Source: CAD feature listing. Evaluate the final solid. Frame: model axes, mm. A direction names the side the tool comes from. Give positions to 0.01 mm unless a question says otherwise; leave off trailing zeros. Order: outer loops, then holes, each group sorted by start corner. A loop starts at its lowest first (then second) coordinate and runs counter-clockwise, first axis right, second up. Notation, with made-up numbers: M 80.5,-18.75 L 89.5,-18.75 A28 ccw 89.5,8.25 Z; hole C 20.25,-22.5 d3. An arc over 180 degrees is marked long. Use CSV: the item, a comma, the result in double quotes. Start each with the question number.
Item 1: Section query A-A on y = 71. Return loops of the section in (x, z), and give its area (3 significant figures).
Item 2: Section query D-D on z = -6. Return loops of the section in (x, y).
Item 3: Ray query, probe 1 along X at (y, z) = (65, 1); probe 2 along Z at (x, y) = (-9, 83.5); probe 3 along Y at (x, z) = (-10, -19.25). Return the intervals inside material, ascending. Write a range as from..to.
Item 4: Section query B-B on z = 1. Return loops of the section in (x, y).
Item 5: Access query for faces 1 (the face through (-12, 62, 0)), 2 (the face through (4.62, 86.46, 1.48)), 3 (the face through (-11.717, 48, 1)). Directions: +Z, -Z, +X, -X, +Y, -Y. A direction counts if a zero-diameter tool reaches every point of the face in a straight line with its end or side. Return the directions, or none.
Item 6: Section query C-C on y = 52. Return loops of the section in (x, z), and give its area (3 significant figures).
Item 7: First-contact query: pin 1 (21 mm diameter, centred on x = -4.66, y = 73.72, fed in from -Z); pin 2 (3.5 mm diameter, centred on y = 46.5, z = 1.5, fed in from -X); pin 3 (8 mm diameter, centred on y = 33, z = -3, fed in from -X); pin 4 (2.5 mm diameter, centred on x = 3.74, y = 82.62, fed in from +Z). Flat tips, straight axial feed; report the tip coordinate or a pass-through.
Item 8: Pull-direction query (X, two-part tool) for faces 4 (the face through (-17.3, 26.26, 1.2)), 5 (the face through (2.42, 52.34, 1.48)), 6 (the face through (-17.61, 85.583, 1.479)); classes: +X half, -X half, draft (parallel to the pull), parting line (faces both ways), or undercut.
from build123d import *

# Parameters (mm, degrees)
SKETCH1_R           = 1
BOSS_EXTRUDE1_DEPTH = 3
SKETCH2_W           = 24
SKETCH2_H           = 3
BOSS_EXTRUDE2_DEPTH = 25
FILLET3_R           = 12
SKETCH3_R           = 1.5
CUT_EXTRUDE1_DEPTH  = 25
FILLET5_R           = 3
FILLET6_R           = 6


with BuildPart() as part:
    # Sketch1 → Boss-Extrude1 (new body)
    with BuildSketch(Plane.XY):
        Polygon((-5.464285714, 44.366071429), (10.535714286, 60.544642857), (10.535714286, 80.544642857), (-1.464285714, 92.544642857), (-33.464285714, 92.544642857), (-45.464285714, 80.544642857), (-45.464285714, 60.544642857), (-29.464285714, 44.366071429), (-29.464285714, 24.544642857), (-5.464285714, 24.544642857), align=None)
        with BuildLine():
            Line((-23.211141689, 41.803891012), (-23.211141689, 53.258480522))
            ThreePointArc((-23.211141689, 53.258480522), (-21.337713702, 55.131908509), (-19.464285714, 53.258480522))
            Line((-19.464285714, 53.258480522), (-19.464285714, 41.803891012))
            ThreePointArc((-19.464285714, 41.803891012), (-21.337713702, 39.930463025), (-23.211141689, 41.803891012))
        make_face(mode=Mode.SUBTRACT)
        with BuildLine():
            ThreePointArc((-15.464285714, 53.258480522), (-13.590857727, 55.131908509), (-11.71742974, 53.258480522))
            Line((-11.71742974, 53.258480522), (-11.71742974, 41.803891012))
            ThreePointArc((-11.71742974, 41.803891012), (-13.590857727, 39.930463025), (-15.464285714, 41.803891012))
            Line((-15.464285714, 41.803891012), (-15.464285714, 53.258480522))
        make_face(mode=Mode.SUBTRACT)
        with Locations((-38.664285714, 64.817850901)):
            Circle(SKETCH1_R, mode=Mode.SUBTRACT)
        with BuildLine():
            ThreePointArc((-24.437255613, 79.199248551), (-17.464285714, 85.584683016), (-10.491315816, 79.199248551))
            ThreePointArc((-10.491315816, 79.199248551), (3.335714286, 73.717850901), (-10.491315816, 68.236453251))
            ThreePointArc((-10.491315816, 68.236453251), (-17.464285714, 61.851018785), (-24.437255613, 68.236453251))
            ThreePointArc((-24.437255613, 68.236453251), (-38.264285714, 73.717850901), (-24.437255613, 79.199248551))
        make_face(mode=Mode.SUBTRACT)
        with Locations((-38.664285714, 82.617850901)):
            Circle(SKETCH1_R, mode=Mode.SUBTRACT)
        with Locations((3.735714286, 64.817850901)):
            Circle(SKETCH1_R, mode=Mode.SUBTRACT)
        with Locations((3.735714286, 82.617850901)):
            Circle(SKETCH1_R, mode=Mode.SUBTRACT)
    extrude(amount=BOSS_EXTRUDE1_DEPTH)

    # Sketch2 → Boss-Extrude2 (add)
    with BuildSketch(Plane(origin=(0, 0, 0), x_dir=(-1, 0, 0), z_dir=(0, 0, -1))):
        with Locations((17.464285714, 26.044642857)):
            Rectangle(SKETCH2_W, SKETCH2_H)
    extrude(amount=BOSS_EXTRUDE2_DEPTH)

    # Fillet3
    fillet3_edges = [part.edges().sort_by_distance(p)[0] for p in [
        (-29.464285714, 26.044642857, -25),
        (-5.464285714, 26.044642857, -25),
    ]]
    fillet(fillet3_edges, radius=FILLET3_R - 0.0001)  # a hair under: the kernel refuses the full size

    # Sketch3 → Cut-Extrude1 (cut)
    with BuildSketch(Plane(origin=(0, 27.544642857, 0), x_dir=(1, 0, 0), z_dir=(0, 1, 0))):
        with Locations(Location((-17.464285714, 12.5, 0), (0, 0, 270))):
            Circle(SKETCH3_R)
        with Locations(Location((-25.464285714, 12.5, 0), (0, 0, 270))):
            Circle(SKETCH3_R)
        with Locations(Location((-9.464285714, 12.5, 0), (0, 0, 180))):
            Circle(SKETCH3_R)
    extrude(amount=-CUT_EXTRUDE1_DEPTH, mode=Mode.SUBTRACT)

    # Fillet5
    fillet5_edges = [part.edges().sort_by_distance(p)[0] for p in [
        (-17.464285714, 27.544642857, 0),
    ]]
    fillet(fillet5_edges, radius=FILLET5_R)

    # Fillet6
    fillet6_edges = [part.edges().sort_by_distance(p)[0] for p in [
        (-17.464285714, 24.544642857, 3),
    ]]
    fillet(fillet6_edges, radius=FILLET6_R)


solid = part.part
Verdict:
1,outline,"M -45.46,0 L -37.79,0 L -37.79,3 L -45.46,3 Z; M 2.86,0 L 10.54,0 L 10.54,3 L 2.86,3 Z"
1,area,"46.1 mm2"
2,outline,"M -29.46,24.54 L -5.46,24.54 L -5.46,27.54 L -29.46,27.54 Z"
3,probe 1,"-45.46..-39.65, -37.68..-23.31, -11.62..2.75, 4.72..10.54"
3,probe 2,"0..3"
3,probe 3,"24.54..27.54"
4,outline,"M -45.46,60.54 L -29.46,44.37 L -29.46,26.07 L -5.46,26.07 L -5.46,44.37 L 10.54,60.54 L 10.54,80.54 L -1.46,92.54 L -33.46,92.54 L -45.46,80.54 Z; hole C -38.66,64.82 d2; hole C -38.66,82.62 d2; hole M -24.44,68.24 A7 ccw -10.49,68.24 A8 ccw long -10.49,79.2 A7 ccw -24.44,79.2 A8 ccw long Z; hole M -23.21,41.8 A1.87 ccw -19.46,41.8 L -19.46,53.26 A1.87 ccw -23.21,53.26 Z; hole M -15.46,41.8 A1.87 ccw -11.72,41.8 L -11.72,53.26 A1.87 ccw -15.46,53.26 Z; hole C 3.74,64.82 d2; hole C 3.74,82.62 d2"
5,face 1,"-Z, +X, -X, +Y"
5,face 2,"+Z, -Z, +X, +Y"
5,face 3,"+Z, -Z"
6,outline,"M -37.01,0 L -23.21,0 L -23.21,3 L -37.01,3 Z; M -19.46,0 L -15.46,0 L -15.46,3 L -19.46,3 Z; M -11.72,0 L 2.09,0 L 2.09,3 L -11.72,3 Z"
6,area,"94.8 mm2"
7,pin 1,"z = 0"
7,pin 2,"x = -33.31"
7,pin 3,"x = -29.46"
7,pin 4,"z = 3"
8,face 4,"draft"
8,face 5,"+X half"
8,face 6,"undercut"
